Geometry: final body of the model. Coordinates: model frame, mm. A direction names the side the tool comes from. Coordinates: 2 decimals unless noted, no trailing zeros. Loops run counter-clockwise (first coordinate to the right, second up) from the corner with the lowest first, then second, coordinate; pieces in that order, holes last. Notation, with made-up numbers: (-21, 4.5) - (4, 4.5) arc R16 cw to (4, 9.5) - close; hole circle Ø3 at (73, 0). An arc over 180 degrees is marked (long way). Put each result on its own line as item: value. Start each with the question number.
1) Section D-D on y = 9. Output: boundary loops of the cut face in (x, z) (1 decimal), and give its area (3 significant figures).
2) Material intervals for line 1 along X through (y, z) = (0, 0.55); line 2 along X through (y, z) = (0, 2.4); line 3 along Y through (x, z) = (0, 2.6), sorted ascending. Write a range as from..to.
3) Section B-B on y = -5. Output: boundary loops of the cut face in (x, z) (1 decimal).
4) Draft query along Y for faces 3 (the cylindrical face through (-0.14, 4.06, 0.5)), 4 (the flat face through (5, 0, 0)), 5 (the cylindrical face through (-3.137, -22.214, 2.898)), 6 (the flat face through (3, -3, 1.016)). Return one class per face: +Y half, -Y half, draft (parallel to the pull), parting line (faces both ways), or undercut.
5) Section C-C on x = 0. Output: boundary loops of the cut face in (y, z) (3 decimals).
6) Reachability of faces 1 (the flat face through (2.667, -16.1, 2.2)), 2 (the flat face through (-16, -5, 5.715)) from +Z, -Z, +X, -X, +Y, -Y: full face, straight path, thin tool, end or side. Return the list, or none.
7) Contact query for flat-ended pins moving along their axis: pin 1 Ø2 at (y, z) = (16, 4.5) entering from +X; pin 2 Ø1.5 at (x, z) = (-5.5, 4) entering from +Y; pin 3 Ø6 at (x, y) = (14.5, -8.5) entering from -Z; pin 4 Ø1.7 at (y, z) = (-11, 2.5) entering from -X. Output: stop coordinate, or through.
8) Section A-A on z = 4.95. Output: boundary loops of the cut face in (x, y), and give its area (3 significant figures).
```python
from build123d import *

# Parameters (mm, degrees)
F1_DEPTH = 1.016
F3_DEPTH = 4.699
F4_R     = 1.27


with BuildPart() as f1:
    # F0 (on Top) → F1 (new body)
    with BuildSketch(Plane.XY):
        with BuildLine():
            ThreePointArc((-2.667, -3.0664649028), (0, 4.064), (2.667, -3.0664649028))
            Line((2.667, -3.0664649028), (2.667, -22.7038919791))
            ThreePointArc((2.667, -22.7038919791), (0, 22.86), (-2.667, -22.7038919791))
            Line((-2.667, -22.7038919791), (-2.667, -3.0664649028))
        make_face()
    extrude(amount=F1_DEPTH)

    # F2 (on face) → F3 (join)
    with BuildSketch(Plane.XY.offset(1.016)):
        with BuildLine():
            ThreePointArc((2.667, -22.7038919791), (17.0813819699, -15.1923003525), (22.86, 0))
            ThreePointArc((22.86, 0), (-15.1923003525, 17.0813819699), (-2.667, -22.7038919791))
            Line((-2.667, -22.7038919791), (-2.667, -15.9069718048))
            ThreePointArc((-2.667, -15.9069718048), (-10.4194193216, 12.3117968632), (16.129, 0))
            ThreePointArc((16.129, 0), (12.3117968632, -10.4194193216), (2.667, -15.9069718048))
            Line((2.667, -15.9069718048), (2.667, -22.7038919791))
        make_face()
    extrude(amount=F3_DEPTH)

    # F4
    f4_edges = [f1.edges().sort_by_distance(p)[0] for p in [
        (-2.667, -22.703892, 2.8575),
        (2.667, -22.703892, 2.8575),
    ]]
    fillet(f4_edges, radius=F4_R)


solid = f1.part
```
Answer block:
1. outline: (-21, 0) - (21, 0) - (21, 5.7) - (13.4, 5.7) - (13.4, 1) - (-13.4, 1) - (-13.4, 5.7) - (-21, 5.7) - close
1. area: 114 mm²
2. line 1: x = -22.86..-4.06, 4.06..22.86
2. line 2: x = -22.86..-16.13, 16.13..22.86
2. line 3: y = 16.13..22.86
3. outline: (-22.3, 0) - (-2.7, 0) - (-2.7, 1) - (-15.3, 1) - (-15.3, 5.7) - (-22.3, 5.7) - close; (2.7, 0) - (22.3, 0) - (22.3, 5.7) - (15.3, 5.7) - (15.3, 1) - (2.7, 1) - close
4. face 3: undercut
4. face 4: draft
4. face 5: -Y half
4. face 6: undercut
5. outline: (4.064, 0) - (22.86, 0) - (22.86, 5.715) - (16.129, 5.715) - (16.129, 1.016) - (4.064, 1.016) - close
6. face 1: +Z, -Z, -Y
6. face 2: +Z, +X, -X, +Y, -Y
7. pin 1: stops at x = 17.25
7. pin 2: stops at y = 22.36
7. pin 3: stops at z = 0
7. pin 4: stops at x = -20.48
8. outline: (-4.17, -22.48) arc R1.27 ccw to (-2.67, -21.23) - (-2.67, -15.91) arc R16.13 cw (long way) to (2.67, -15.91) - (2.67, -21.23) arc R1.27 ccw to (4.17, -22.48) arc R22.86 ccw (long way) to start
8. area: 787 mm²
